Work out the finished part from the listing and answer in its coordinate system (mm). Face numbers are marked on the shaded views. A direction names the side the tool comes from. Round coordinates to 2 decimals unless told otherwise and drop trailing zeros. Write each loop counter-clockwise with the first axis right and the second up, starting at its lowest first coordinate (ties: lowest second). Pieces come first, ordered by that corner, then holes. Notation, with made-up numbers: M 76,5 L 99,5 A21 ccw 99,14 Z; hole C -6,22 d6. An arc over 180 degrees is marked long. One line per item, written item: value. Start each with the question number.
Q1. Find section A-A (z = 7.75). Write down the section's boundary in (x, y).
Q2. The mould has two halves that part along Y. Classify the marked faces 5, 6 and 7: released by +Y, released by -Y, zero draft, split by the parting line, or undercut.
Q3. A tool of negligible diameter and unlimited length cuts with its end or side. For the marked faces 1, 2, 3 and 4, from which of +Z, -Z, +X, -X, +Y, -Y can it reach the whole face along a straight path? Write none if from no direction.
Q4. Find section B-B (x = 0). Write down the section's boundary in (y, z), and give its area (3 significant figures).
Q5. Consider probe 1 along Y at (x, z) = (0, 2.95); probe 2 along Z at (x, y) = (8.25, -5.5); probe 3 along X at (y, z) = (4, 0.5). Determine where each line is inside the solid, lowest interval first.
Q6. Find section C-C (y = -4.5). Write down the section's boundary in (x, z).
Q7. Given pin 1 Ø1.1 at (x, z) = (4, 1.5) entering from -Y; pin 2 Ø4 at (x, y) = (5.5, 0) entering from +Z; pin 3 Ø1 at (x, z) = (5, 6) entering from +Y; pin 4 Ø2 at (y, z) = (0.5, 2.5) entering from -X, each flat-ended and moving along its own axis, determine where each tip first touches the part or whether it passes through.
Q8. Find section D-D (x = -6.25). Write down the section's boundary in (y, z), and give its area (3 significant figures).
from build123d import *

# Parameters (mm, degrees)
SKETCH1_R           = 10
SKETCH1_R_2         = 5
BOSS_EXTRUDE2_DEPTH = 4
BOSS_EXTRUDE3_DEPTH = 4
SKETCH3_W           = 3
SKETCH3_H           = 2
BOSS_EXTRUDE4_DEPTH = 4


with BuildPart() as part:
    # Sketch1 → Boss-Extrude2 (new body)
    with BuildSketch(Plane.XY):
        Circle(SKETCH1_R)
        Circle(SKETCH1_R_2, mode=Mode.SUBTRACT)
    extrude(amount=BOSS_EXTRUDE2_DEPTH)

    # Sketch2 → Boss-Extrude3 (add)
    with BuildSketch(Plane.XY.offset(4)):
        with BuildLine():
            ThreePointArc((-5.5, 0), (-5.449982192, 0.74006358), (-5.300838508, 1.466666667))
            Line((-5.300838508, 1.466666667), (-9.155993787, 2.533333333))
            ThreePointArc((-9.155993787, 2.533333333), (-9.413605605, 1.278291639), (-9.5, 0))
            ThreePointArc((-9.5, 0), (-9.413605605, -1.278291639), (-9.155993787, -2.533333333))
            Line((-9.155993787, -2.533333333), (-5.300838508, -1.466666667))
            ThreePointArc((-5.300838508, -1.466666667), (-5.449982192, -0.74006358), (-5.5, 0))
        make_face()
        with BuildLine():
            ThreePointArc((3.920589846, -3.857327476), (2.75, -4.763139721), (1.380248662, -5.323994143))
            Line((1.380248662, -5.323994143), (2.38406587, -9.195989883))
            ThreePointArc((2.38406587, -9.195989883), (4.75, -8.227241336), (6.771927916, -6.66265655))
            Line((6.771927916, -6.66265655), (3.920589846, -3.857327476))
        make_face()
        with BuildLine():
            Line((2.38406587, 9.195989883), (1.380248662, 5.323994143))
            ThreePointArc((1.380248662, 5.323994143), (2.75, 4.763139721), (3.920589846, 3.857327476))
            Line((3.920589846, 3.857327476), (6.771927916, 6.66265655))
            ThreePointArc((6.771927916, 6.66265655), (4.75, 8.227241336), (2.38406587, 9.195989883))
        make_face()
    extrude(amount=BOSS_EXTRUDE3_DEPTH)

    # Sketch3 → Boss-Extrude4 (add)
    with BuildSketch(Plane(origin=(0, 0, 0), x_dir=(-1, 0, 0), z_dir=(0, 0, -1))):
        with Locations((-5, 0)):
            Rectangle(SKETCH3_W, SKETCH3_H)
    extrude(amount=-BOSS_EXTRUDE4_DEPTH)


solid = part.part
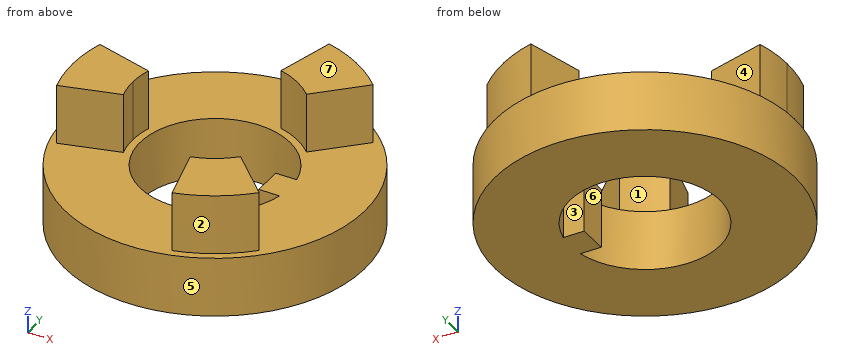
The answers:
1. outline: M -9.16,-2.53 L -5.3,-1.47 A5.5 cw -5.3,1.47 L -9.16,2.53 A9.5 ccw Z; M 1.38,-5.32 L 2.38,-9.2 A9.5 ccw 6.77,-6.66 L 3.92,-3.86 A5.5 cw Z; M 1.38,5.32 A5.5 cw 3.92,3.86 L 6.77,6.66 A9.5 ccw 2.38,9.2 Z
2. face 5: split by the parting line
2. face 6: undercut
2. face 7: zero draft
3. face 1: +Z, -X
3. face 2: +Z, +X, -Y
3. face 3: +Z, -Z
3. face 4: +Z, +X, +Y
4. outline: M -10,0 L -5,0 L -5,4 L -10,4 Z; M 5,0 L 10,0 L 10,4 L 5,4 Z
4. area: 40.0 mm2
5. probe 1: -10 to -5, 5 to 10
5. probe 2: 0 to 4
5. probe 3: -9.17 to -3, 3 to 9.17
6. outline: M -8.93,0 L -2.18,0 L -2.18,4 L -8.93,4 Z; M 2.18,0 L 8.93,0 L 8.93,4 L 4.57,4 L 4.57,8 L 3.16,8 L 3.16,4 L 2.18,4 Z
7. pin 1: y = -9.39
7. pin 2: z = 4
7. pin 3: y = 8.37
7. pin 4: x = -10
8. outline: M -7.81,0 L 7.81,0 L 7.81,4 L 1.73,4 L 1.73,8 L -1.73,8 L -1.73,4 L -7.81,4 Z
8. area: 76.3 mm2
